Geometry check sheet. Reference: drawing and pictorial views, mm from the part's lowest x, y, z. A direction names the side the tool comes from. Give positions to 0.01 mm unless a question says otherwise; leave off trailing zeros. Write each loop counter-clockwise with the first axis right and the second up, starting at its lowest first coordinate (ties: lowest second). Pieces come first, ordered by that corner, then holes. Notation, with made-up numbers: (27.5, 13.25) - (31.5, 13.25) arc R24 cw to (31.5, 34.25) - close; hole circle Ø7 at (42.5, 89.25). An arc over 180 degrees is marked (long way). Put each result on its own line as item: value.
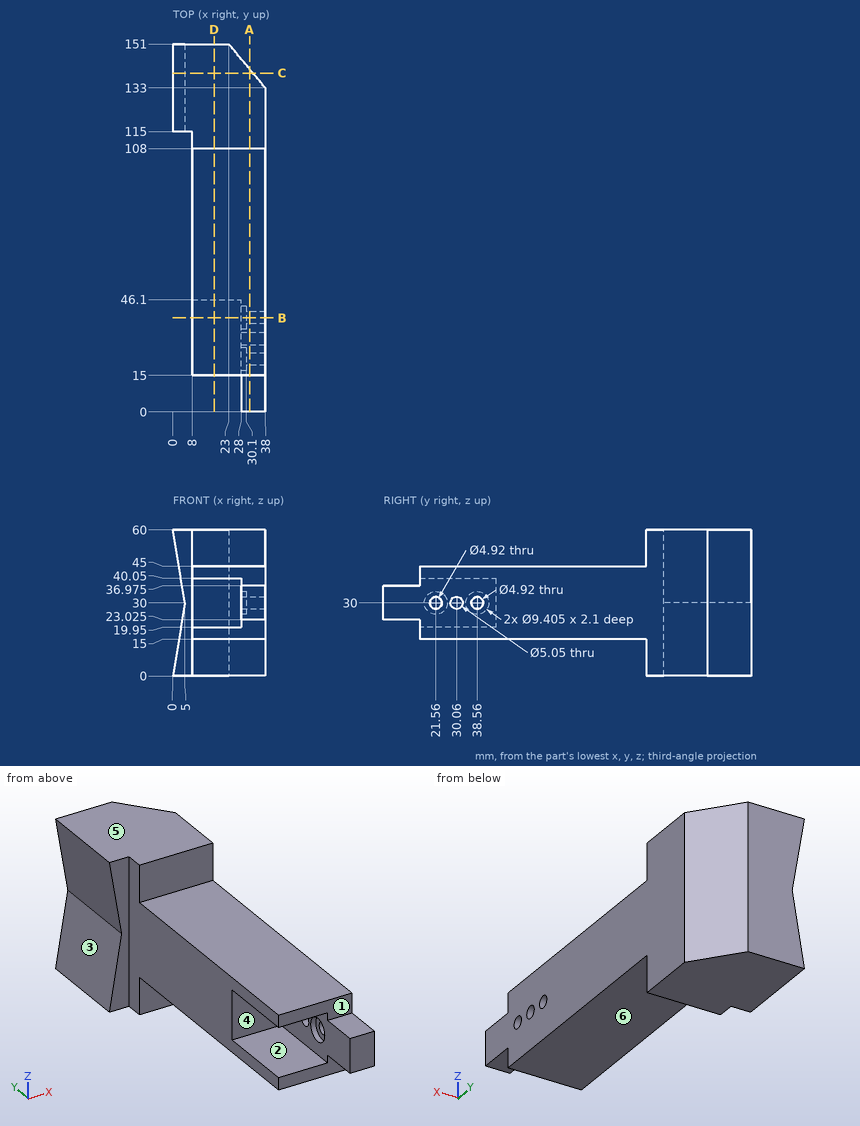
Q1. Set-up check for the marked faces 1, 2 and 3: record each of +Z, -Z, +X, -X, +Y, -Y from which the full face is reachable in a straight line by a thin tool's end or side.
Answers follow:
face 1: +Z, +X, -X, -Y
face 2: -X, -Y
face 3: -X, +Y, -Y
Q2. Section check D-D, the plane x = 17. Record the cut outline in (y, z), plus the area to 3 significant figures.
Answers follow:
outline: (15, 15) - (108, 15) - (108, 0) - (151, 0) - (151, 60) - (108, 60) - (108, 45) - (15, 45) - (15, 40.05) - (46.1, 40.05) - (46.1, 19.95) - (15, 19.95) - close
area: 4,740 mm2
Q3. Go/stop test with flat-tipped pins: pin 1 Ø4.5 at (y, z) = (21.56, 30) entering from -X; pin 2 Ø4.5 at (y, z) = (21, 32) entering from -X; pin 3 Ø1 at (x, z) = (25.5, 48.5) entering from +Y; pin 4 Ø16 at (x, y) = (19, 26) entering from -Z. Record where each tip stops, or that it passes through.
Answers follow:
pin 1: passes through
pin 2: stops at x = 30.1
pin 3: stops at y = 148.6
pin 4: stops at z = 15
Q4. Scan lines: line 1 along Y through (x, z) = (28.7, 30) (1 decimal); line 2 along Z through (x, y) = (29, 21); line 3 along Y through (x, z) = (34, 30) (3 decimals). Record each from-to range of solid material in increasing order.
Answers follow:
line 1: y = 0 to 16.9, 26.3 to 27.5, 32.6 to 33.9, 43.3 to 144.2
line 2: z = 15 to 25.33, 34.67 to 45
line 3: y = 0 to 19.1, 24.02 to 27.535, 32.585 to 36.1, 41.02 to 137.8
Q5. Section check B-B, the plane y = 38.56. Record the cut outline in (x, z).
Answers follow:
outline: (8, 15) - (38, 15) - (38, 27.54) - (30.1, 27.54) - (30.1, 25.3) - (28, 25.3) - (28, 19.95) - (8, 19.95) - close; (8, 40.05) - (28, 40.05) - (28, 34.7) - (30.1, 34.7) - (30.1, 32.46) - (38, 32.46) - (38, 45) - (8, 45) - close
Q6. Release check for a two-part mould opening along Z. For the marked faces 4, 5 and 6 record: released by +Z, released by -Z, zero draft, split by the parting line, or undercut.
Answers follow:
face 4: undercut
face 5: released by +Z
face 6: released by -Z
Q7. Section check A-A, the plane x = 31.5. Record the cut outline in (y, z) (3 decimals).
Answers follow:
outline: (0, 23.025) - (15, 23.025) - (15, 15) - (108, 15) - (108, 0) - (140.8, 0) - (140.8, 60) - (108, 60) - (108, 45) - (15, 45) - (15, 36.975) - (0, 36.975) - close; hole circle Ø4.92 at (21.56, 30); hole circle Ø5.05 at (30.06, 30); hole circle Ø4.92 at (38.56, 30)
Q8. Section check C-C, the plane y = 139. Record the cut outline in (x, z).
Answers follow:
outline: (0, 0) - (33, 0) - (33, 60) - (0, 60) - (5, 30) - close
